Input: part model. Units: mm. Frame: model coordinates. A direction names the side the tool comes from. Round coordinates to 2 decimals unless told otherwise and drop trailing zeros. Write item = value, one per line. Start each with the question number.
```python
from build123d import *

# Parameters (mm, degrees)
F0_W     = 1219.2
F0_H     = 76.2
F1_DEPTH = 12.7
F2_W     = 31.75
F2_H     = 6.35
F3_DEPTH = 76.2
F4_DEPTH = 76.2
F5_W     = 31.75
F5_H     = 6.35
F6_DEPTH = 9.525
F7_DEPTH = 9.525


with BuildPart() as f1:
    # F0 (on Top) → F1 (new body, symmetric)
    with BuildSketch(Plane.XY):
        Rectangle(F0_W, F0_H)
    extrude(amount=F1_DEPTH, both=True)

    # F2 (on face) → F3 (cut, through all)
    with BuildSketch(Plane.XZ.offset(38.1)):
        with Locations((-355.6, 0)):
            Rectangle(F2_W, F2_H)
    extrude(amount=-F3_DEPTH, mode=Mode.SUBTRACT)

    # F2 (on face) → F4 (cut, through all)
    with BuildSketch(Plane.XZ.offset(38.1)):
        with Locations((355.6, 0)):
            Rectangle(F2_W, F2_H)
    extrude(amount=-F4_DEPTH, mode=Mode.SUBTRACT)

    # F5 (on face) → F6 (cut, through all)
    with BuildSketch(Plane.XY.offset(12.7)):
        with Locations((-355.6, 34.925)):
            Rectangle(F5_W, F5_H)
    extrude(amount=-F6_DEPTH, mode=Mode.SUBTRACT)

    # F5 (on face) → F7 (cut, through all)
    with BuildSketch(Plane.XY.offset(12.7)):
        with Locations((355.6, 34.925)):
            Rectangle(F5_W, F5_H)
    extrude(amount=-F7_DEPTH, mode=Mode.SUBTRACT)


solid = f1.part
```
1. Reachability of faces 1 (the flat face through (-9, -38.1, 0)), 2 (the flat face through (355, -1, -3.175)) from +Z, -Z, +X, -X, +Y, -Y: full face, straight path, thin tool, end or side. Return the list, or none.
2. Line query: line 1 along X through (y, z) = (-0.5, -0.75) (3 decimals); line 2 along Z through (x, y) = (345.5, -14.5) (3 decimals). Output: solid intervals per line, ascending.
3. Mould query, pull axis Z, two halves, no side actions, for faces 3 (the flat face through (-9, 38.1, 0)), 4 (the flat face through (-9, 1, 12.7)), 5 (the flat face through (355, -4, 3.175)). Classes: pulls with the +Z half, pulls with the -Z half, needs draft (parallel to the pull), parting line crosses it, or undercut.
4. Pin query (flat end, axial travel): P1, Ø5, axis at x = 362, z = 10, coming from the +Y side. Return the tip coordinate at first contact, or that it passes through.
Check sheet entries:
q1.face_1 = +Z, -Z, +X, -X, -Y
q1.face_2 = +Y, -Y
q2.line_1 = -609.6 to -371.475, -339.725 to 339.725, 371.475 to 609.6
q2.line_2 = -12.7 to -3.175, 3.175 to 12.7
q3.face_3 = needs draft
q3.face_4 = pulls with the +Z half
q3.face_5 = undercut
q4.P1 = 31.75
